Check sheet for the modelled part. Datum: model origin and axes. Units: mm. Face numbers are marked on the shaded views. A direction names the side the tool comes from. Coordinates: 2 decimals unless noted, no trailing zeros. Loops run counter-clockwise (first coordinate to the right, second up) from the corner with the lowest first, then second, coordinate; pieces in that order, holes last. Notation, with made-up numbers: M -16,17 L -3,17 A24 cw -3,32 Z; hole C -25.75,77 d8. An arc over 180 degrees is marked long. Write each question's results on one line, items separated by ' | '. Start each with the question number.
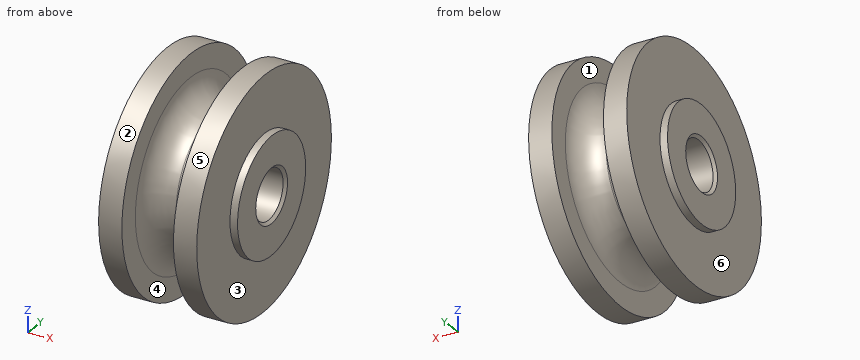
from build123d import *
from build123d import SkipClean  # not in build123d's __all__

# Parameters (mm, degrees)
F3_SIZE = 0.5


with BuildPart() as f1:
    # F0 (on Front) → F1 (revolve)
    with BuildSketch(Plane.XZ):
        with BuildLine():
            Line((0, 4.4), (10.1, 4.4))
            Line((10.1, 4.4), (10.1, 10.5))
            Line((10.1, 10.5), (8.75, 10.5))
            Line((8.75, 10.5), (8.75, 20.75))
            Line((8.75, 20.75), (4.6, 20.75))
            Line((4.6, 20.75), (4.6, 16.6))
            ThreePointArc((4.6, 16.6), (3.2526911935, 13.3473088065), (0, 12))
            Line((0, 12), (0, 4.4))
        make_face()
    revolve(axis=Axis((5.05, 0, 0), (1, 0, 0)))

    # F2: F1 across plane


with BuildPart() as f1_1:
    add(f1.part, clean=False)
    with SkipClean():  # cleaning this boolean's faces spoils the solid; the shape is the same uncleaned
        add(f1.part.mirror(Plane.YZ), clean=False)

    # F3
    f3_edges = [f1_1.edges().sort_by_distance(p)[0] for p in [
        (10.1, 0, -4.4),
        (-10.1, 0, -4.4),
    ]]
    chamfer(f3_edges, length=F3_SIZE)


solid = f1_1.part
1) Set-up check for the marked faces 5 and 6: record each of +Z, -Z, +X, -X, +Y, -Y from which the full face is reachable in a straight line by a thin tool's end or side.
2) Section check B-B (x = -5.5). Enter the section's corners in (y, z), then the cut area to 3 significant figures.
3) Section check C-C (x = 3.25). Enter the section's corners in (y, z), then the cut area to 3 significant figures.
4) Section check A-A (y = -17.5). Enter the section's corners in (x, z).
5) Thickness scan on probe 1 along X at (y, z) = (-1, 17.5); probe 2 along Y at (x, z) = (7.25, 0). Record the ranges inside material, lowest first.
6) Release check for a two-part mould opening along X. For the marked faces 1, 2, 3 and 4 record: +X half, -X half, draft (parallel to the pull), parting line (faces both ways), or undercut.
7) Gauge pin test, flat ends, axial feed: P1, Ø10, axis at y = 13, z = -10, coming from the -X side; P2, Ø6, axis at x = -7, y = -11, coming from the +Z side; P3, Ø5, axis at x = 7, z = 3.5, coming from the +Y side; P4, Ø5.5, axis at y = 0, z = 0, coming from the -X side. Record the tip position at first contact, or that the pin passes through.
Return value:
1) face 5: +X, -X | face 6: -X
2) outline: C 0,0 d41.5; hole C 0,0 d8.8 | area: 1,290 mm2
3) outline: C 0,0 d26.69; hole C 0,0 d8.8 | area: 499 mm2
4) outline: M -8.75,-11.15 L -4.6,-11.15 L -4.6,11.15 L -8.75,11.15 Z; M 4.6,-11.15 L 8.75,-11.15 L 8.75,11.15 L 4.6,11.15 Z
5) probe 1: x = -8.75 to -4.6, 4.6 to 8.75 | probe 2: y = -20.75 to -4.4, 4.4 to 20.75
6) face 1: undercut | face 2: draft | face 3: +X half | face 4: undercut
7) P1: stops at x = -8.75 | P2: stops at z = 19.15 | P3: stops at y = 20.73 | P4: passes through
